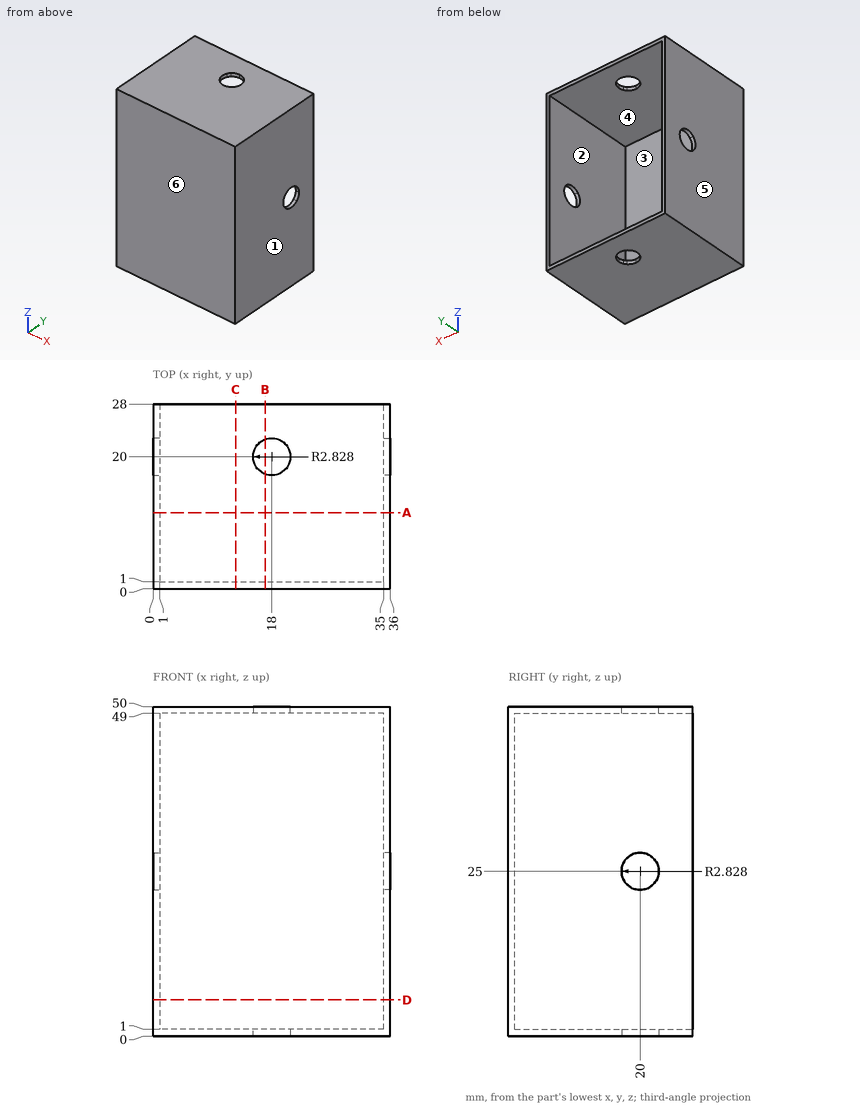
Geometry check sheet. Reference: drawing and pictorial views, mm from the part's lowest x, y, z. A direction names the side the tool comes from. Give positions to 0.01 mm unless a question says otherwise; leave off trailing zeros. Order: outer loops, then holes, each group sorted by start corner. A loop starts at its lowest first (then second) coordinate and runs counter-clockwise, first axis right, second up.
1. Thickness scan on L1, parallel to X at y = 8.25, z = 39; L2, parallel to Z at x = 4, y = 13.75; L3, parallel to Y at x = 3, z = 40. Record the ranges inside material, lowest first.
2. Release check for a two-part mould opening along X. For the marked faces 3, 4, 5 and 6 record: pulls with the +X half, pulls with the -X half, needs draft (parallel to the pull), parting line crosses it, or undercut.
3. Section check D-D, the plane z = 5.5. Enter the section's corners in (x, y).
4. Section check A-A, the plane y = 11.5. Enter the section's corners in (x, z).
5. Section check B-B, the plane x = 17. Enter the section's corners in (y, z) (1 decimal).
6. Access from +Z, -Z, +X, -X, +Y, -Y to the whole of each face (thin tool, end or side, straight path). Record for the marked faces 1 and 2.
7. Section check C-C, the plane x = 12.5. Enter the section's corners in (y, z).
8. Gauge pin test, flat ends, axial feed: pin 1 Ø6 at (x, z) = (27.5, 27.5) entering from -Y; pin 2 Ø17 at (x, z) = (16, 20.5) entering from +Y. Record the tip position at first contact, or that the pin passes through.
Values follow:
1. L1: x = 0 to 1, 35 to 36
1. L2: z = 0 to 1, 49 to 50
1. L3: y = 0 to 1
2. face 3: undercut
2. face 4: undercut
2. face 5: pulls with the -X half
2. face 6: needs draft
3. outline: (0, 0) - (36, 0) - (36, 28) - (35, 28) - (35, 1) - (1, 1) - (1, 28) - (0, 28) - close
4. outline: (0, 0) - (36, 0) - (36, 50) - (0, 50) - close; hole (1, 1) - (35, 1) - (35, 49) - (1, 49) - close
5. outline: (0, 0) - (17.4, 0) - (17.4, 1) - (1, 1) - (1, 49) - (17.4, 49) - (17.4, 50) - (0, 50) - close; (22.6, 0) - (28, 0) - (28, 1) - (22.6, 1) - close; (22.6, 49) - (28, 49) - (28, 50) - (22.6, 50) - close
6. face 1: +Z, -Z, +X, +Y, -Y
6. face 2: +Y
7. outline: (0, 0) - (28, 0) - (28, 1) - (1, 1) - (1, 49) - (28, 49) - (28, 50) - (0, 50) - close
8. pin 1: stops at y = 0
8. pin 2: stops at y = 1
